Answer from the drawing. Dimensions are ordinates in mm from the lowest x, y and z of the part. Give positions to 0.01 mm unless a question says otherwise; leave off trailing zeros. Loops run counter-clockwise (first coordinate to the right, second up) from the corner with the lowest first, then second, coordinate; pieces in that order, holes last.
(1) Find section C-C, the plane y = 8.89. Write down the section's boundary in (x, z).
(2) Find section B-B, the plane z = 1.05. State how many separate pieces and enclosed holes the cut face has, then the cut area to 3 significant figures.
(3) Find section A-A, the plane x = 15.24. Write down the section's boundary in (y, z).
(4) Straight lines are drawn through the part: probe 1 along X at (y, z) = (8.75, 0.5); probe 2 along Y at (x, z) = (18, 1.6); probe 3 along X at (y, z) = (8, 0.5) (1 decimal). For each, find the intervals that lie inside material, in ascending order.
(5) This flat-tipped pin is pushed along its axis until it touches: P1, Ø2, axis at x = 2.54, y = 8.89, coming from the -Z side. Where does it stop, or does it pass through?
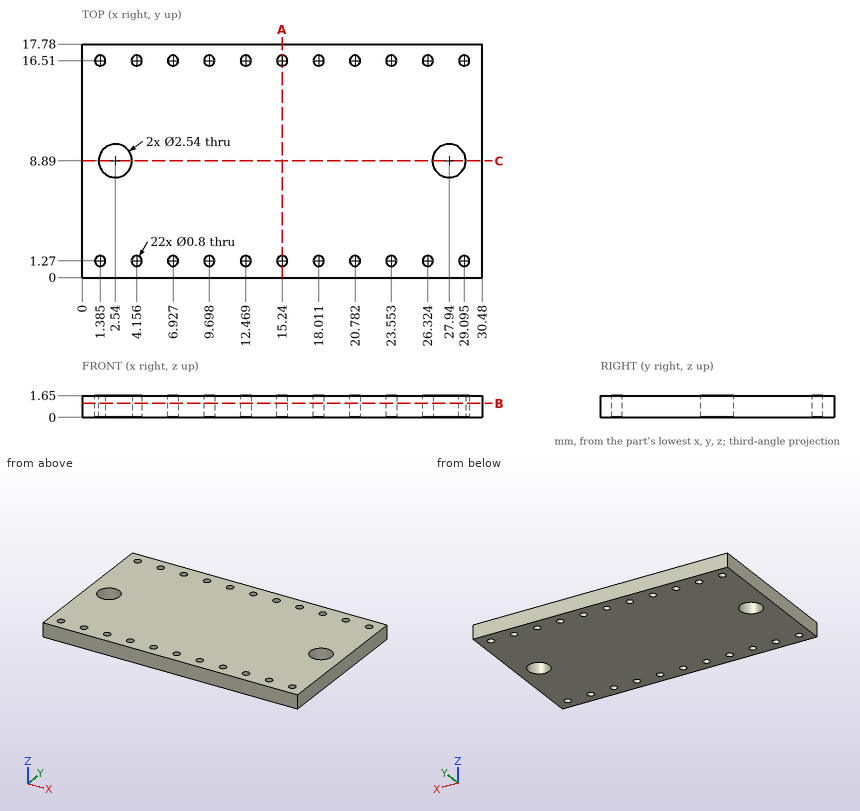
Entries:
1. outline: (0, 0) - (1.27, 0) - (1.27, 1.65) - (0, 1.65) - close; (3.81, 0) - (26.67, 0) - (26.67, 1.65) - (3.81, 1.65) - close; (29.21, 0) - (30.48, 0) - (30.48, 1.65) - (29.21, 1.65) - close
2. separate pieces: 1
2. enclosed holes: 24
2. area: 521 mm2
3. outline: (0, 0) - (0.87, 0) - (0.87, 1.65) - (0, 1.65) - close; (1.67, 0) - (16.11, 0) - (16.11, 1.65) - (1.67, 1.65) - close; (16.91, 0) - (17.78, 0) - (17.78, 1.65) - (16.91, 1.65) - close
4. probe 1: x = 0 to 1.28, 3.8 to 26.68, 29.2 to 30.48
4. probe 2: y = 0 to 0.87, 1.67 to 16.11, 16.91 to 17.78
4. probe 3: x = 0 to 1.6, 3.4 to 27, 28.8 to 30.5
5. P1: passes through
